Part model, mm, in its own coordinate system. A direction names the side the tool comes from. Round coordinates to 2 decimals unless told otherwise and drop trailing zeros. Order: outer loops, then holes, each group sorted by start corner. A loop starts at its lowest first (then second) coordinate and runs counter-clockwise, first axis right, second up. Notation, with made-up numbers: (68.5, -11) -> (125.5, -11) arc R14 cw to (125.5, 11) -> close; hole circle Ø1 at (-11.75, 59.5). An arc over 180 degrees is marked (long way). Use CSV: the item, a comma, the result in double quotes.
```python
from build123d import *

# Parameters (mm, degrees)
F1_DEPTH = 18.7
F2_W     = 13
F2_H     = 12
F3_DEPTH = 15
F4_R     = 1.5
F5_DEPTH = 5
F4_R_2   = 1
F6_DEPTH = 6
F4_R_3   = 2
F7_DEPTH = 0.8


with BuildPart() as f1:
    # F0 (on Right) → F1 (new body)
    with BuildSketch(Plane.YZ):
        with BuildLine():
            Line((4.905354, 6), (-4.905354, 6))
            ThreePointArc((-4.905354, 6), (-7.75, 0), (-4.905354, -6))
            Line((-4.905354, -6), (4.905354, -6))
            ThreePointArc((4.905354, -6), (7.75, 0), (4.905354, 6))
        make_face()
    extrude(amount=F1_DEPTH)

    # F2 (on face) → F3 (join)
    with BuildSketch(Plane.YZ.offset(18.7)):
        Rectangle(F2_W, F2_H)
    extrude(amount=F3_DEPTH)

    # F4 (on face) → F5 (join)
    with BuildSketch(Plane.YZ.offset(33.7)):
        Circle(F4_R)
    extrude(amount=F5_DEPTH)

    # F4 (on face) → F6 (cut)
    with BuildSketch(Plane.YZ.offset(33.7)):
        with Locations((-4.5, 0)):
            Circle(F4_R_2)
        with Locations((4.5, 0)):
            Circle(F4_R_2)
    extrude(amount=-F6_DEPTH, mode=Mode.SUBTRACT)

    # F4 (on face) → F7 (join)
    with BuildSketch(Plane.YZ.offset(33.7)):
        Circle(F4_R_3)
        Circle(F4_R, mode=Mode.SUBTRACT)
    extrude(amount=F7_DEPTH)


solid = f1.part
```
(1) Cut at C-C, the plane x = 31. Give the cut face in (y, z), then the cut area to 3 significant figures.
Reply:
outline,"(-6.5, -6) -> (6.5, -6) -> (6.5, 6) -> (-6.5, 6) -> close; hole circle Ø2 at (-4.5, 0); hole circle Ø2 at (4.5, 0)"
area,"150 mm2"
(2) Drop flat-ended pins along their axis: P1, Ø3, axis at x = 29, z = -1, coming from the +Y side; P2, Ø6, axis at x = 25, z = 0, coming from the -Y side; P3, Ø1.8, axis at y = 4.5, z = 0, coming from the +X side. Give the stop position or say it passes through.
Reply:
P1,"y = 6.5"
P2,"y = -6.5"
P3,"x = 27.7"
(3) Which spindle directions (+Z, -Z, +X, -X, +Y, -Y) get a long thin tool onto all of the face, cutting with end or side? Do faces 4 (the face through (18.7, -6.1, 5.5)), 5 (the face through (9.22, -7.75, 0.1)), 6 (the face through (18.7, 6, -5.5)). Say none if no direction does.
Reply:
face 4,"+Z, -X, -Y"
face 5,"-X, -Y"
face 6,"-Z, -X, +Y"
(4) Cut at A-A, the plane z = 0. Give the cut face in (x, y), then the cut area to 3 significant figures.
Reply:
outline,"(0, -7.75) -> (18.7, -7.75) -> (18.7, -6.5) -> (33.7, -6.5) -> (33.7, -5.5) -> (27.7, -5.5) -> (27.7, -3.5) -> (33.7, -3.5) -> (33.7, -2) -> (34.5, -2) -> (34.5, -1.5) -> (38.7, -1.5) -> (38.7, 1.5) -> (34.5, 1.5) -> (34.5, 2) -> (33.7, 2) -> (33.7, 3.5) -> (27.7, 3.5) -> (27.7, 5.5) -> (33.7, 5.5) -> (33.7, 6.5) -> (18.7, 6.5) -> (18.7, 7.75) -> (0, 7.75) -> close"
area,"477 mm2"
(5) Cut at B-B, the plane y = 0. Give the cut face in (x, z).
Reply:
outline,"(0, -6) -> (33.7, -6) -> (33.7, -2) -> (34.5, -2) -> (34.5, -1.5) -> (38.7, -1.5) -> (38.7, 1.5) -> (34.5, 1.5) -> (34.5, 2) -> (33.7, 2) -> (33.7, 6) -> (0, 6) -> close"
(6) Cut at D-D, the plane x = 23. Give the cut face in (y, z).
Reply:
outline,"(-6.5, -6) -> (6.5, -6) -> (6.5, 6) -> (-6.5, 6) -> close"
(7) Pull direction Y, two halves, no side cores. Call faces 1 (the face through (30.7, 3.5, 0)), 2 (the face through (18.7, 6, 5.5)), 3 (the face through (34, 0, -2)): released by +Y, released by -Y, zero draft, split by the parting line, or undercut.
Reply:
face 1,"undercut"
face 2,"zero draft"
face 3,"split by the parting line"
(8) Probe probe 1 along Z at (x, y) = (30.35, -4.5); probe 2 along Y at (x, z) = (30.5, 0.75); probe 3 along Y at (x, z) = (25.5, -1). List the from-to ranges inside material, lowest first. Write a range as [from, to].
Reply:
probe 1,"[-6, -1], [1, 6]"
probe 2,"[-6.5, -5.16], [-3.84, 3.84], [5.16, 6.5]"
probe 3,"[-6.5, 6.5]"
